from build123d import *

# Parameters (mm, degrees)
SKETCH1_R           = 44
BOSS_EXTRUDE1_DEPTH = 4
SKETCH2_R           = 3.5
CUT_EXTRUDE1_DEPTH  = 2
SKETCH3_R           = 1
CUT_EXTRUDE2_DEPTH  = 63.353829072
SKETCH5_R           = 1.5
CUT_EXTRUDE3_DEPTH  = 63.257529665
SKETCH6_R           = 1.5
CUT_EXTRUDE4_DEPTH  = 63.353829072
FILLET1_R           = 2


with BuildPart() as part:
    # Sketch1 → Boss-Extrude1 (new body)
    with BuildSketch(Plane(origin=(0, 0, 0), x_dir=(1, 0, 0), z_dir=(0, 1, 0))):
        with Locations(Location((0, 0, 0), (0, 0, 270))):
            Circle(SKETCH1_R)
    extrude(amount=BOSS_EXTRUDE1_DEPTH)

    # Sketch2 → Cut-Extrude1 (cut)
    with BuildSketch(Plane(origin=(0, 4, 0), x_dir=(1, 0, 0), z_dir=(0, 1, 0))):
        with Locations(Location((0, 0, 0), (0, 0, 270))):
            Circle(SKETCH2_R)
    extrude(amount=-CUT_EXTRUDE1_DEPTH, mode=Mode.SUBTRACT)

    # Sketch3 → Cut-Extrude2 (cut, through all)
    with BuildSketch(Plane(origin=(0, 4, 0), x_dir=(1, 0, 0), z_dir=(0, 1, 0))):
        with Locations(Location((0, 13.5, 0), (0, 0, 270))):
            Circle(SKETCH3_R)
        with Locations(Location((0, -13.5, 0), (0, 0, 90))):
            Circle(SKETCH3_R)
        with Locations(Location((-13.5, 0, 0), (0, 0, 270))):
            Circle(SKETCH3_R)
        with Locations(Location((13.5, 0, 0), (0, 0, 90))):
            Circle(SKETCH3_R)
    extrude(amount=-CUT_EXTRUDE2_DEPTH, mode=Mode.SUBTRACT)

    # Sketch5 → Cut-Extrude3 (cut, through all)
    with BuildSketch(Plane(origin=(0, 2, 0), x_dir=(1, 0, 0), z_dir=(0, 1, 0))):
        with Locations(Location((0, 0, 0), (0, 0, 270))):
            Circle(SKETCH5_R)
    extrude(amount=-CUT_EXTRUDE3_DEPTH, mode=Mode.SUBTRACT)

    # Sketch6 → Cut-Extrude4 (cut, through all)
    with BuildSketch(Plane(origin=(0, 4, 0), x_dir=(1, 0, 0), z_dir=(0, 1, 0))):
        with Locations(Location((-9.899494937, 9.899494937, 0), (0, 0, 270))):
            Circle(SKETCH6_R)
        with Locations(Location((9.899494937, -9.899494937, 0), (0, 0, 90))):
            Circle(SKETCH6_R)
    extrude(amount=-CUT_EXTRUDE4_DEPTH, mode=Mode.SUBTRACT)

    # Fillet1
    fillet1_edges = [part.edges().sort_by_distance(p)[0] for p in [
        (0, 4, -44),
    ]]
    fillet(fillet1_edges, radius=FILLET1_R)


solid = part.part
Verification items for the finished model (mm, model axes). A direction names the side the tool comes from. Round coordinates to 2 decimals unless told otherwise and drop trailing zeros. Write each loop counter-clockwise with the first axis right and the second up, starting at its lowest first coordinate (ties: lowest second). Pieces come first, ordered by that corner, then holes.
(1) Depth check by flat-ended pin: pin 1 Ø1.5 at (x, y) = (9, 1.5) entering from +Z; pin 2 Ø1.5 at (y, z) = (1.5, 21) entering from +X; pin 3 Ø6.5 at (x, z) = (0, 0) entering from +Y. Enter the tip coordinate at first touch or a pass-through.
Returned:
pin 1: stops at z = 43.22
pin 2: stops at x = 39.06
pin 3: stops at y = 2
(2) Material ranges on line 1 (X direction, y = 1.45, z = 0); line 2 (X direction, y = 2.6, z = 0); line 3 (X direction, y = 3.2, z = 13), recorded low to high.
Returned:
line 1: x = -44 to -14.5, -12.5 to -1.5, 1.5 to 12.5, 14.5 to 44
line 2: x = -43.91 to -14.5, -12.5 to -3.5, 3.5 to 12.5, 14.5 to 43.91
line 3: x = -41.62 to -0.87, 0.87 to 41.62
(3) Section check C-C (y = 0.95). Enter the section's corners in (x, z).
Returned:
outline: circle Ø88 at (0, 0); hole circle Ø2 at (-13.5, 0); hole circle Ø3 at (-9.9, -9.9); hole circle Ø3 at (0, 0); hole circle Ø2 at (0, -13.5); hole circle Ø2 at (0, 13.5); hole circle Ø3 at (9.9, 9.9); hole circle Ø2 at (13.5, 0)
(4) Access from +Z, -Z, +X, -X, +Y, -Y to the whole of each face (thin tool, end or side, straight path). Record for faces 5 (the flat face through (0, 2, 2)), 6 (the cylindrical face through (-8.635, 2.028, -9.093)).
Returned:
face 5: +Y
face 6: +Y, -Y
(5) Section check A-A (z = 0). Enter the section's corners in (x, y).
Returned:
outline: (-44, 0) - (-14.5, 0) - (-14.5, 4) - (-42, 4) arc R2 ccw to (-44, 2) - close; (-12.5, 0) - (-1.5, 0) - (-1.5, 2) - (-3.5, 2) - (-3.5, 4) - (-12.5, 4) - close; (1.5, 0) - (12.5, 0) - (12.5, 4) - (3.5, 4) - (3.5, 2) - (1.5, 2) - close; (14.5, 0) - (44, 0) - (44, 2) arc R2 ccw to (42, 4) - (14.5, 4) - close
(6) Mould release check, pull along X, two halves, no side actions. Record for faces 1 (the flat face through (1, 4, 9)), 2 (the cylindrical face through (14.476, 2.028, 0.217)), 3 (the cylindrical face through (-3.417, 3.014, -0.759)), 4 (the cylindrical face through (-42.954, 0.986, -9.538)): pulls with the +X half, pulls with the -X half, needs draft (parallel to the pull), parting line crosses it, or undercut.
Returned:
face 1: needs draft
face 2: undercut
face 3: undercut
face 4: parting line crosses it
(7) Section check B-B (x = 0). Enter the section's corners in (y, z), plus the area to 3 significant figures.
Returned:
outline: (0, -44) - (2, -44) arc R2 ccw to (4, -42) - (4, -14.5) - (0, -14.5) - close; (0, -12.5) - (4, -12.5) - (4, -3.5) - (2, -3.5) - (2, -1.5) - (0, -1.5) - close; (0, 1.5) - (2, 1.5) - (2, 3.5) - (4, 3.5) - (4, 12.5) - (0, 12.5) - close; (0, 14.5) - (4, 14.5) - (4, 42) arc R2 ccw to (2, 44) - (0, 44) - close
area: 314 mm2
